```python
from build123d import *

# Parameters (mm, degrees)
SKETCH1_R           = 100
SKETCH1_R_2         = 60
BOSS_EXTRUDE1_DEPTH = 5


with BuildPart() as part:
    # Sketch1 → Boss-Extrude1 (new body)
    with BuildSketch(Plane(origin=(0, 0, 0), x_dir=(1, 0, 0), z_dir=(0, 1, 0))):
        Circle(SKETCH1_R)
        Circle(SKETCH1_R_2, mode=Mode.SUBTRACT)
        with BuildLine():
            Line((0, 61.5), (-50, 61.5))
            ThreePointArc((-50, 61.5), (-51.5, 63), (-50, 64.5))
            Line((-50, 64.5), (0, 64.5))
            ThreePointArc((0, 64.5), (1.5, 63), (0, 61.5))
        make_face(mode=Mode.SUBTRACT)
        with BuildLine():
            Line((36.148793016, 49.754545154), (-4.302056703, 79.143807769))
            ThreePointArc((-4.302056703, 79.143807769), (-4.633904316, 81.239011139), (-2.538700946, 81.570858752))
            Line((-2.538700946, 81.570858752), (37.912148773, 52.181596137))
            ThreePointArc((37.912148773, 52.181596137), (38.243996386, 50.086392767), (36.148793016, 49.754545154))
        make_face(mode=Mode.SUBTRACT)
        with BuildLine():
            Line((58.489975752, 19.004545154), (43.039126033, 66.557370969))
            ThreePointArc((43.039126033, 66.557370969), (44.002185316, 68.447481235), (45.892295582, 67.484421952))
            Line((45.892295582, 67.484421952), (61.343145301, 19.931596137))
            ThreePointArc((61.343145301, 19.931596137), (60.380086018, 18.041485871), (58.489975752, 19.004545154))
        make_face(mode=Mode.SUBTRACT)
        with BuildLine():
            Line((58.489975752, -19.004545154), (73.940825471, 28.548280661))
            ThreePointArc((73.940825471, 28.548280661), (75.830935737, 29.511339944), (76.79399502, 27.621229678))
            Line((76.79399502, 27.621229678), (61.343145301, -19.931596137))
            ThreePointArc((61.343145301, -19.931596137), (59.453035035, -20.89465542), (58.489975752, -19.004545154))
        make_face(mode=Mode.SUBTRACT)
        with BuildLine():
            Line((36.148793016, -49.754545154), (76.599642735, -20.365282539))
            ThreePointArc((76.599642735, -20.365282539), (78.694846105, -20.697130153), (78.362998492, -22.792333523))
            Line((78.362998492, -22.792333523), (37.912148773, -52.181596137))
            ThreePointArc((37.912148773, -52.181596137), (35.816945403, -51.849748524), (36.148793016, -49.754545154))
        make_face(mode=Mode.SUBTRACT)
        with BuildLine():
            Line((0, -61.5), (50, -61.5))
            ThreePointArc((50, -61.5), (51.5, -63), (50, -64.5))
            Line((50, -64.5), (0, -64.5))
            ThreePointArc((0, -64.5), (-1.5, -63), (0, -61.5))
        make_face(mode=Mode.SUBTRACT)
        with BuildLine():
            Line((-36.148793016, -49.754545154), (4.302056703, -79.143807769))
            ThreePointArc((4.302056703, -79.143807769), (4.633904316, -81.239011139), (2.538700946, -81.570858752))
            Line((2.538700946, -81.570858752), (-37.912148773, -52.181596137))
            ThreePointArc((-37.912148773, -52.181596137), (-38.243996386, -50.086392767), (-36.148793016, -49.754545154))
        make_face(mode=Mode.SUBTRACT)
        with BuildLine():
            Line((-58.489975752, -19.004545154), (-43.039126033, -66.557370969))
            ThreePointArc((-43.039126033, -66.557370969), (-44.002185316, -68.447481235), (-45.892295582, -67.484421952))
            Line((-45.892295582, -67.484421952), (-61.343145301, -19.931596137))
            ThreePointArc((-61.343145301, -19.931596137), (-60.380086018, -18.041485871), (-58.489975752, -19.004545154))
        make_face(mode=Mode.SUBTRACT)
        with BuildLine():
            Line((-58.489975752, 19.004545154), (-73.940825471, -28.548280661))
            ThreePointArc((-73.940825471, -28.548280661), (-75.830935737, -29.511339944), (-76.79399502, -27.621229678))
            Line((-76.79399502, -27.621229678), (-61.343145301, 19.931596137))
            ThreePointArc((-61.343145301, 19.931596137), (-59.453035035, 20.89465542), (-58.489975752, 19.004545154))
        make_face(mode=Mode.SUBTRACT)
        with BuildLine():
            Line((-36.148793016, 49.754545154), (-76.599642735, 20.365282539))
            ThreePointArc((-76.599642735, 20.365282539), (-78.694846105, 20.697130153), (-78.362998492, 22.792333523))
            Line((-78.362998492, 22.792333523), (-37.912148773, 52.181596137))
            ThreePointArc((-37.912148773, 52.181596137), (-35.816945403, 51.849748524), (-36.148793016, 49.754545154))
        make_face(mode=Mode.SUBTRACT)
    extrude(amount=BOSS_EXTRUDE1_DEPTH)


solid = part.part
```
Can you work these out from the model? Positions are in its coordinate system, mm. Coordinates: 2 decimals unless noted, no trailing zeros. Order: outer loops, then holes, each group sorted by start corner. A loop starts at its lowest first (then second) coordinate and runs counter-clockwise, first axis right, second up. Notation, with made-up numbers: (-13, -33.75) - (35, -33.75) arc R23 cw to (35, -3.75) - close; hole circle Ø9 at (22, 47). An arc over 180 degrees is marked (long way). Answer in a Markdown table with one row per item.
1. Suppose I cut it at C-C (y = 3.65). Give the number of separate pieces and of enclosed holes in the cut face, and give its area (3 significant figures).
Reply:
| item | result |
|---|---|
| separate pieces | 1 |
| enclosed holes | 11 |
| area | 18,500 mm^2 |
2. Suppose I cut it at B-B (x = -25.5). Please give me the cut outline in (y, z), and give its area (3 significant figures).
Reply:
| item | result |
|---|---|
| outline | (0, -96.69) - (5, -96.69) - (5, -64.5) - (0, -64.5) - close; (0, -61.5) - (5, -61.5) - (5, -54.31) - (0, -54.31) - close; (0, 54.31) - (5, 54.31) - (5, 57.49) - (0, 57.49) - close; (0, 61.2) - (5, 61.2) - (5, 96.69) - (0, 96.69) - close |
| area | 390 mm^2 |
3. For pin 1 (2 mm diameter, centred on x = 79, y = 2.5, fed in from -Z); pin 2 (1 mm diameter, centred on y = 1.5, z = 54.5, fed in from -X), each with a flat end and sliding along its axis, tell me the tip position at first contact or that it passes through.
Reply:
| item | result |
|---|---|
| pin 1 | stops at z = -62.58 |
| pin 2 | stops at x = -84.17 |
4. If we mould it in two halves opening along X, with no side actions, what happens to faces 1 (the flat face through (43, 0, 43)), 2 (the flat face through (66.107, 2.465, -4.439))? For each: pulls with the +X half, pulls with the -X half, needs draft (parallel to the pull), parting line crosses it, or undercut.
Reply:
| item | result |
|---|---|
| face 1 | needs draft |
| face 2 | undercut |
5. If I drill on line 1 along X through (y, z) = (3.6, 0); line 2 along Z through (x, y) = (0, 1.45); line 3 along X through (y, z) = (1.75, -11), over which ranges is the centre line in solid material (lowest first)?
Reply:
| item | result |
|---|---|
| line 1 | x = -100 to -67.82, -64.66 to -60, 60 to 64.66, 67.82 to 100 |
| line 2 | z = -100 to -79.73, -76.02 to -64.5, -61.5 to -60, 60 to 61.5, 64.5 to 76.02, 79.73 to 100 |
| line 3 | x = -99.39 to -64.25, -61.09 to -58.98, 58.98 to 68.24, 71.39 to 99.39 |
6. Suppose I cut it at A-A (z = 0). Please give me the cut outline in (x, y).
Reply:
| item | result |
|---|---|
| outline | (-100, 0) - (-67.82, 0) - (-67.82, 5) - (-100, 5) - close; (-64.66, 0) - (-60, 0) - (-60, 5) - (-64.66, 5) - close; (60, 0) - (64.66, 0) - (64.66, 5) - (60, 5) - close; (67.82, 0) - (100, 0) - (100, 5) - (67.82, 5) - close |
